CAD build for the part. Positions are in the model's coordinates, mm. Coordinates: 2 decimals unless noted, no trailing zeros. Loops run counter-clockwise (first coordinate to the right, second up) from the corner with the lowest first, then second, coordinate; pieces in that order, holes last. Notation, with made-up numbers: M 70,39.25 L 111,39.25 A10 cw 111,50.25 Z; hole C 52.25,25 d2. An arc over 180 degrees is marked long. Answer as a JSON object with one key per item and string values. Group by question number.
```python
from build123d import *

# Parameters (mm, degrees)
SALIENTE_EXTRUIR1_DEPTH = 8.77
SALIENTE_EXTRUIR2_START = 25.9
CROQUIS2_R              = 2.5
SALIENTE_EXTRUIR2_DEPTH = 25.9
SALIENTE_EXTRUIR6_START = 10
CROQUIS3_R              = 2.5
SALIENTE_EXTRUIR6_DEPTH = 10
CORTAR_EXTRUIR1_DEPTH   = 10


with BuildPart() as part:
    # Croquis1 → Saliente-Extruir1 (new body)
    with BuildSketch(Plane.XY):
        with BuildLine():
            Line((-53.549500652, 10.469715541), (-53.549500652, 11.069715541))
            Line((-53.549500652, 11.069715541), (-52.649500652, 11.069715541))
            Line((-52.649500652, 11.069715541), (-52.649500652, 10.469715541))
            ThreePointArc((-52.649500652, 10.469715541), (-53.099500652, 5.510549015), (-53.549500652, 10.469715541))
        make_face()
    extrude(amount=SALIENTE_EXTRUIR1_DEPTH)

    # Croquis2 → Saliente-Extruir2 (add)
    with BuildSketch(Plane(origin=(0, 0, 0), x_dir=(-1, 0, 0), z_dir=(0, 0, -1)).offset(SALIENTE_EXTRUIR2_START)):
        with Locations((53.099500652, 8.010549015)):
            Circle(CROQUIS2_R)
    extrude(amount=-SALIENTE_EXTRUIR2_DEPTH)

    # Croquis3 → Saliente-Extruir6 (add)
    with BuildSketch(Plane(origin=(0, 0, -25.9), x_dir=(-1, 0, 0), z_dir=(0, 0, -1)).offset(SALIENTE_EXTRUIR6_START)):
        with Locations((53.099500652, 8.010549015)):
            Circle(CROQUIS3_R)
    extrude(amount=-SALIENTE_EXTRUIR6_DEPTH)

    # Croquis8 → Cortar-Extruir1 (cut)
    with BuildSketch(Plane(origin=(0, 0, -35.9), x_dir=(-1, 0, 0), z_dir=(0, 0, -1))):
        with BuildLine():
            Line((52.649500652, 6.15138249), (52.649500652, 5.55138249))
            ThreePointArc((52.649500652, 5.55138249), (53.099500652, 5.510549014), (53.549500652, 5.55138249))
            Line((53.549500652, 5.55138249), (53.549500652, 6.15138249))
            Line((53.549500652, 6.15138249), (52.649500652, 6.15138249))
        make_face()
    extrude(amount=-CORTAR_EXTRUIR1_DEPTH, mode=Mode.SUBTRACT)


solid = part.part
```
Item 1: Slice it at C-C, the plane z = -18. Write the cut outline in (x, y).
Item 2: Pin check, flat tips, straight feed: pin 1 (1.5 mm diameter, centred on y = 6, z = -7, fed in from +X); pin 2 (1 mm diameter, centred on x = -53.5, z = -17.5, fed in from +Y). Stop position of each tip, or through.
Item 3: Slice it at A-A, the plane x = -51. Write the cut outline in (y, z).
Item 4: Pull direction X, two halves, no side cores. Call faces 1 (the cylindrical face through (-54.634, 9.984, -13.878)), 2 (the flat face through (-53, 8, -35.9)), 3 (the flat face through (-53, 6.151, -31)): released by +X, released by -X, zero draft, split by the parting line, or undercut.
Item 5: Drill centre lines: L1, parallel to Y at x = -53.1, z = -29.5; L2, parallel to X at y = 8.1, z = -19.5; L3, parallel to Y at x = -53.3, z = -0.5. Where is each one in solid material? Low to high. Write a range as from..to.
Item 6: Slice it at B-B, the plane z = -27.5. Write the cut outline in (x, y).
Computed:
{
 "1": {"outline": "C -53.1,8.01 d5"},
 "2": {"pin 1": "x = -50.94", "pin 2": "y = 10.51"},
 "3": {"outline": "M 6.65,-35.9 L 9.37,-35.9 L 9.37,8.77 L 6.65,8.77 Z"},
 "4": {"face 1": "split by the parting line", "face 2": "zero draft", "face 3": "undercut"},
 "5": {"L1": "6.15..10.51", "L2": "-55.6..-50.6", "L3": "5.52..10.5"},
 "6": {"outline": "M -53.55,5.55 L -53.55,6.15 L -52.65,6.15 L -52.65,5.55 A2.5 ccw long Z"}
}
